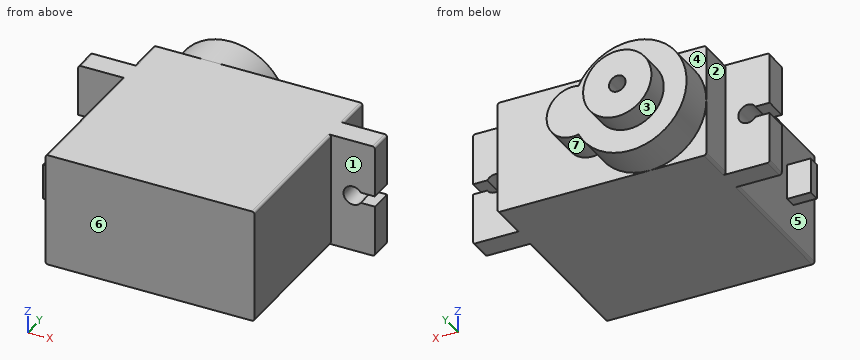
Autodesk Inventor part; units mm, degrees
ref_plane "Work Plane1" through (0, 18.2372, 0) normal (0, 1, 0) x (1, 0, 0)
ref_plane "Work Plane2" through (11.2141, 0, 12.2428) normal (1, 0, 0) x (0, 0, -1)
ref_plane "YZ Plane" through (0, 0, 0) normal (1, 0, 0) x (0, 1, 0)
sketch "Sketch1" plane through (0, 0, 0) normal (0, 0, 1) x (1, 0, 0)
  line L0 (0, 0) -> (22.4282, 0)
  line L1 (22.4282, 0) -> (22.4282, 22.225)
  line L2 (22.4282, 22.225) -> (0, 22.225)
  line L3 (0, 22.225) -> (0, 0)
  dimension "d0" = 22.4282
  dimension "d1" = 22.225
extrude "Extrusion1" add sketch "Sketch1" along normal blind 12.2428
ref_plane "Work Plane1" through (0, 18.2372, 0) normal (0, 1, 0) x (1, 0, 0)
sketch "Sketch2" plane through (0, 18.2372, 0) normal (0, 1, 0) x (1, 0, 0)
  line L0 (22.4282, -12.2428) -> (27.1526, -12.2428)
  line L1 (27.1526, 0) -> (22.4282, 0)
  line L2 (22.4282, 0) -> (22.4282, -12.2428)
  arc A0 (25.6304, -5.5499) -> (25.6304, -6.6929) centre (24.7904, -6.1214) ccw
  line L3 (22.4282, 0) -> (22.4282, -12.2428)
  line L4 (25.6304, -6.6929) -> (27.1526, -6.6929)
  line L5 (25.6304, -5.5499) -> (27.1526, -5.5499)
  line L6 (27.1526, -12.2428) -> (27.1526, -6.6929)
  line L7 (27.1526, -5.5499) -> (27.1526, 0)
  point P0 (0, 0)
  point P1 (22.4282, -6.1214)
  point P2 (24.7904, 0)
  point P3 (27.1526, -6.1214)
  dimension "d6" = 2.032
  dimension "d23" = 1.143
  dimension "d24" = 0.5715
  dimension "d25" = 4.7244
extrude "Extrusion2" add sketch "Sketch2" against normal blind 2.4892
ref_plane "Work Plane2" through (11.2141, 0, 12.2428) normal (1, 0, 0) x (0, 0, -1)
mirror "Mirror1" about plane through (11.2141, 0, 12.2428) normal (1, 0, 0) of "Extrusion2"
sketch "Sketch3" plane through (0, 22.225, 0) normal (0, 1, 0) x (1, 0, 0)
  arc A0 (11.6052, -3.4011) -> (11.6052, -8.8417) centre (6.1214, -6.1214) ccw
  line L0 (22.4282, 0) -> (0, 0)
  line L1 (0, 0) -> (0, -12.2428)
  line L2 (22.4282, -12.2428) -> (0, -12.2428)
  arc A1 (11.6052, -8.8417) -> (11.6052, -3.4011) centre (12.2428, -6.1214) ccw
  dimension "d9" = 5.588
extrude "Extrusion3" add sketch "Sketch3" along normal blind 4.064 contours A1 A0
sketch "Sketch4" plane through (0, 26.289, 0) normal (0, 1, 0) x (1, 0, 0)
  arc A0 (6.1214, -12.2428) -> (11.6052, -8.8417) centre (6.1214, -6.1214) ccw
  circle A1 centre (6.1214, -6.1214) radius 3.6703
  circle A2 centre (6.1214, -6.1214) radius 0.889
  point P0 (0, 0)
  dimension "d12" = 7.3406
  dimension "d15" = 1.778
extrude "Extrusion4" add sketch "Sketch4" along normal blind 2.54
sketch "Sketch5" plane through (0, 0, 0) normal (-1, 0, 0) x (0, 0, 1)
  circle A0 centre (4.8514, 4.953) radius 0.635
  circle A1 centre (6.1214, 4.953) radius 0.635
  circle A2 centre (7.3914, 4.953) radius 0.635
  line L0 (4.8514, 4.318) -> (7.3914, 4.318) construction
  line L1 (0, 0) -> (12.2428, 0)
  point P0 (6.1214, 0)
  point P1 (6.7564, 4.953)
  point P2 (5.4864, 4.953)
  dimension "d17" = 1.27
  dimension "d18" = 1.27
  dimension "d16" = 1.27
  dimension "d19" = 4.318
extrude "Extrusion5" add sketch "Sketch5" along normal blind 2.54
fillet "Fillet1" radius 0.254 12 edges at (22.4282, 7.874, 0) (22.4282, 20.2311, 0) (22.4282, 20.2311, 12.2428) (22.4282, 7.874, 12.2428) (27.1526, 16.9926, 12.2428) (27.1526, 16.9926, 0) (-4.7244, 16.9926, 0) (-4.7244, 16.9926, 12.2428) (0, 7.874, 12.2428) (0, 7.874, 0) (0, 20.2311, 0) (0, 20.2311, 12.2428)
sketch "Sketch6" plane through (-2.54, 4.953, 4.8514) normal (-1, 0, 0) x (0, 0, 1)
  circle A0 centre (0, 0) radius 0.635
  circle A1 centre (2.54, 0) radius 0.635
  line L0 (-0.635, 0.635) -> (3.175, 0.635)
  line L1 (3.175, 0.635) -> (3.175, -0.635)
  line L2 (3.175, -0.635) -> (-0.635, -0.635)
  line L3 (-0.635, -0.635) -> (-0.635, 0.635)
  circle A2 centre (0, 0) radius 0.635
  circle A3 centre (2.54, 0) radius 0.635
  point P0 (-4.8514, -4.953)
  point P1 (0.635, 0)
  point P2 (1.905, 0)
extrude "Extrusion6" add sketch "Sketch6" against normal up to surface (2.54 mm away)
equation "\"d17\" = d16"
equation "\"d18\" = d16"
properties part number "Servo"
The listing builds one solid part. Answer for the finished solid, in the listing's coordinates (mm). Face numbers are marked on the shaded views. A direction names the side the tool comes from. Coordinates: 2 decimals unless noted, no trailing zeros. Write each loop counter-clockwise with the first axis right and the second up, starting at its lowest first coordinate (ties: lowest second). Pieces come first, ordered by that corner, then holes. Notation, with made-up numbers: M 64,36.5 L 85,36.5 A20 ccw 85,67.5 Z; hole C 9.5,81 d10. An arc over 180 degrees is marked long. Put each result on its own line as item: value. Start each with the question number.
1. A cutting plane is placed at C-C on z = 11.25. Write down the section's boundary in (x, y) (3 decimals).
2. A cutting plane is placed at B-B on x = 3. Write down the section's boundary in (y, z) (3 decimals).
3. Flat-ended cylindrical pins translate along their axes: P1, Ø3, axis at x = -1, z = 5.5, coming from the -Y side; P2, Ø1.5, axis at x = 25.5, z = 7.5, coming from the +Y side; P3, Ø2.5, axis at x = -3, z = 5.5, coming from the -Y side; P4, Ø1, axis at y = 25, z = 4.5, coming from the +X side. Find the tip coordinate at first contact, or state that the pin passes through.
4. Which of the six approach directions +Z, -Z, +X, -X, +Y, -Y give full straight-line access (tool end or side, diameter ignored) to the marked faces 1, 2, 3 and 4?
5. A cutting plane is placed at A-A on y = 10. Write down the section's boundary in (x, z), then the cut area to 3 significant figures.
6. A cutting plane is placed at D-D on x = 13.5. Write down the section's boundary in (y, z) (3 decimals), then the cut area to 3 significant figures.
7. Consider line 1 (X direction, y = 13.5, z = 11.25); line 2 (Y direction, x = 20, z = 10) (3 decimals); line 3 (Y direction, x = 5.5, z = 0.5). Determine where each line is inside the solid, lowest interval first. Write a range as from..to.
8. For a pull along Y with two mould halves and no side action, classify the marked faces 5, 6 and 7 as pulls with the +Y half, pulls with the -Y half, needs draft (parallel to the pull), parting line crosses it, or undercut.
Resolved:
1. outline: M -4.724,15.748 L 0,15.748 L 0,0 L 22.428,0 L 22.428,15.748 L 27.153,15.748 L 27.153,18.237 L 22.428,18.237 L 22.428,22.225 L 9.463,22.225 L 9.463,26.289 L 2.779,26.289 L 2.779,22.225 L 0,22.225 L 0,18.237 L -4.724,18.237 Z
2. outline: M 0,0 L 22.225,0 L 22.225,0.856 L 26.289,0.856 L 26.289,4.191 L 28.829,4.191 L 28.829,8.052 L 26.289,8.052 L 26.289,11.387 L 22.225,11.387 L 22.225,12.243 L 0,12.243 Z
3. P1: stops at y = 0
3. P2: stops at y = 18.24
3. P3: stops at y = 4.32
3. P4: stops at x = 14.8
4. face 1: +Z, -Z, +X, -Y
4. face 2: +Z, -Z, -X, +Y
4. face 3: +Y
4. face 4: +Z, -X, +Y
5. outline: M 0,0.25 A0.25 ccw 0.25,0 L 22.17,0 A0.25 ccw 22.43,0.25 L 22.43,11.99 A0.25 ccw 22.17,12.24 L 0.25,12.24 A0.25 ccw 0,11.99 Z
5. area: 275 mm2
6. outline: M 0,0 L 22.225,0 L 22.225,3.626 L 26.289,3.626 L 26.289,8.617 L 22.225,8.617 L 22.225,12.243 L 0,12.243 Z
6. area: 292 mm2
7. line 1: x = 0..22.43
7. line 2: y = 0..22.225
7. line 3: y = 0..26.29
8. face 5: undercut
8. face 6: pulls with the -Y half
8. face 7: needs draft
